Geometry: final body of the model. Coordinates: model frame, mm. A direction names the side the tool comes from. Give positions to 0.01 mm unless a question says otherwise; leave off trailing zeros. Order: outer loops, then holes, each group sorted by start corner. A loop starts at its lowest first (then second) coordinate and runs counter-clockwise, first axis right, second up. Notation, with made-up numbers: (68, 39) -> (80, 39) arc R21 ccw to (80, 48) -> close; hole circle Ø1 at (-20, 76). An arc over 180 degrees is marked (long way). Answer in a Markdown table with one row per item. Add a question column.
Q1. Cut plane B-B on z = -16.5. Return the cut outline in (x, y).
Q2. Set-up query: faces 4 (the face through (-21.5, -5, 27)), 5 (the face through (0, -10, 0)), 6 (the face through (-23, -5, 22)), 7 (the face through (21.5, -5, -27)). Return all of +Z, -Z, +X, -X, +Y, -Y with unobstructed straight access to the full face (end or side cutting, diameter ignored); none if empty.
Q3. Pull-direction query (X, two-part tool) for faces 1 (the face through (23, -5, -22)), 2 (the face through (24.5, -5, -26)), 3 (the face through (-11.3, -4.9, 41)); classes: +X half, -X half, draft (parallel to the pull), parting line (faces both ways), or undercut.
Q4. Cut plane C-C on x = -11.5. Return the cut outline in (y, z), and give its area (3 significant figures).
Q5. Contact query for flat-ended pins moving along their axis: P1, Ø3.5, axis at x = -23, y = -2.5, coming from the -Z side; P2, Ø3, axis at y = -6.5, z = -0.5, coming from the +X side; P3, Ø1, axis at x = -5.5, y = -4.5, coming from the +Z side; P4, Ø1, axis at x = -3.5, z = -18, coming from the -Y side. Output: stop coordinate, or through.
Q6. Cut plane A-A on y = -4.5. Return the cut outline in (x, z), and give its area (3 significant figures).
Q7. Line query: line 1 along X through (y, z) = (-6.25, 31); line 2 along X through (y, z) = (-3, -28.5); line 3 along X through (y, z) = (-1.75, 5.5). Output: solid intervals per line, ascending. Write a range as from..to.
from build123d import *

# Parameters (mm, degrees)
PAD_DEPTH = 10


with BuildPart() as part:
    # Sketch → Pad (new body)
    with BuildSketch(Plane.XZ):
        with BuildLine():
            Line((-21.5, 31), (-21.5, 22))
            Line((-21.5, 22), (-24.5, 22))
            Line((-24.5, 22), (-24.5, 31))
            ThreePointArc((1.5, 31), (-11.5, 44), (-24.5, 31))
            Line((1.5, 31), (1.5, -31))
            ThreePointArc((1.5, -31), (11.5, -41), (21.5, -31))
            Line((21.5, -31), (21.5, -22))
            Line((21.5, -22), (24.5, -22))
            Line((24.5, -22), (24.5, -31))
            ThreePointArc((-1.5, -31), (11.5, -44), (24.5, -31))
            Line((-1.5, 31), (-1.5, -31))
            ThreePointArc((-1.5, 31), (-11.5, 41), (-21.5, 31))
        make_face()
    extrude(amount=PAD_DEPTH)


solid = part.part
Completed:
| question | item | result |
|---|---|---|
| 1 | outline | (-1.5, -10) -> (1.5, -10) -> (1.5, 0) -> (-1.5, 0) -> close |
| 2 | face 4 | -Z, +Y, -Y |
| 2 | face 5 | +Z, -Z, +X, -X, -Y |
| 2 | face 6 | -Z, -X, +Y, -Y |
| 2 | face 7 | +Z, +Y, -Y |
| 3 | face 1 | draft |
| 3 | face 2 | +X half |
| 3 | face 3 | undercut |
| 4 | outline | (-10, 41) -> (0, 41) -> (0, 44) -> (-10, 44) -> close |
| 4 | area | 30.0 mm² |
| 5 | P1 | stops at z = 22 |
| 5 | P2 | stops at x = 1.5 |
| 5 | P3 | stops at z = 42.78 |
| 5 | P4 | passes through |
| 6 | outline | (-24.5, 22) -> (-21.5, 22) -> (-21.5, 31) arc R10 cw to (-1.5, 31) -> (-1.5, -31) arc R13 ccw to (24.5, -31) -> (24.5, -22) -> (21.5, -22) -> (21.5, -31) arc R10 cw to (1.5, -31) -> (1.5, 31) arc R13 ccw to (-24.5, 31) -> close |
| 6 | area | 457 mm² |
| 7 | line 1 | x = -24.5..-21.5, -1.5..1.5 |
| 7 | line 2 | x = -1.5..1.5, 21.5..24.5 |
| 7 | line 3 | x = -1.5..1.5 |
